The listing builds one solid part. Answer for the finished solid, in the listing's coordinates (mm). Coordinates: 2 decimals unless noted, no trailing zeros. Order: outer loops, then holes, each group sorted by start corner. A loop starts at its lowest first (then second) coordinate and runs counter-clockwise, first axis right, second up. Notation, with made-up numbers: (-23.75, 62.5) -> (-10.75, 62.5) arc R4 ccw to (-10.75, 67.5) -> close; hole circle Ø5 at (-15, 24). An arc over 180 degrees is marked (long way). Answer in a Markdown table with one row per item.
```python
from build123d import *

# Parameters (mm, degrees)
F1_DEPTH = 30


with BuildPart() as f1:
    # F0 (on Top) → F1 (new body)
    with BuildSketch(Plane.XY):
        with BuildLine():
            Line((17.858347, -1.59188), (0, -1.59188))
            Line((0, -1.59188), (0, -17.782362))
            Line((0, -17.782362), (2.289595, -17.782362))
            ThreePointArc((2.289595, -17.782362), (12.923538, -12.427261), (17.858347, -1.59188))
        make_face()
        with BuildLine():
            Line((24.029288, -1.59188), (17.858347, -1.59188))
            ThreePointArc((17.858347, -1.59188), (12.923538, -12.427261), (2.289595, -17.782362))
            Line((2.289595, -17.782362), (24.029288, -17.782362))
            Line((24.029288, -17.782362), (24.029288, -1.59188))
        make_face()
        with BuildLine():
            Line((0, -17.782362), (0, -1.59188))
            Line((0, -1.59188), (17.858347, -1.59188))
            ThreePointArc((17.858347, -1.59188), (17.911445, -0.796727), (17.929156, 0))
            ThreePointArc((17.929156, 0), (-13.463008, 11.840696), (2.289595, -17.782362))
            Line((2.289595, -17.782362), (0, -17.782362))
        make_face()
    extrude(amount=F1_DEPTH)


solid = f1.part
```
(1) For a pull along Y with two mould halves and no side action, classify faces 1 (the flat face through (13, -17.782, 15)), 2 (the flat face through (3, 0, 0)), 3 (the cylindrical face through (-13.054, 12.29, 14.79)), 4 (the cylindrical face through (17.91, -0.81, 14.79)) as released by +Y, released by -Y, zero draft, split by the parting line, or undercut.
Check values:
| item | result |
|---|---|
| face 1 | released by -Y |
| face 2 | zero draft |
| face 3 | split by the parting line |
| face 4 | undercut |
(2) Flat-ended cylindrical pins translate along their axes: pin 1 (6 mm diameter, centred on x = -6.5, z = 23.5, fed in from +Y); pin 2 (2 mm diameter, centred on x = -4.5, y = -3.5, fed in from -Z); pin 3 (17.5 mm diameter, centred on x = 14.5, z = 18, fed in from -Y); pin 4 (1 mm diameter, centred on x = -3.5, z = 16, fed in from +Y). Find the tip coordinate at first contact, or state that the pin passes through.
Check values:
| item | result |
|---|---|
| pin 1 | y = 17.58 |
| pin 2 | z = 0 |
| pin 3 | y = -17.78 |
| pin 4 | y = 17.68 |
(3) A cutting plane is placed at B-B, the plane x = 15. Determine the outline of the cut face in (y, z).
Check values:
| item | result |
|---|---|
| outline | (-17.78, 0) -> (9.82, 0) -> (9.82, 30) -> (-17.78, 30) -> close |
(4) A cutting plane is placed at A-A, the plane z = 19.5. Determine the outline of the cut face in (x, y), then the cut area to 3 significant figures.
Check values:
| item | result |
|---|---|
| outline | (2.29, -17.78) -> (24.03, -17.78) -> (24.03, -1.59) -> (17.86, -1.59) arc R17.93 ccw to (17.93, 0) arc R17.93 ccw (long way) to start |
| area | 1,180 mm² |
(5) A cutting plane is placed at C-C, the plane y = 9. Determine the outline of the cut face in (x, z), then the cut area to 3 significant figures.
Check values:
| item | result |
|---|---|
| outline | (-15.51, 0) -> (15.51, 0) -> (15.51, 30) -> (-15.51, 30) -> close |
| area | 930 mm² |
(6) Find the intervals of material crossed by line 1 along Y through (x, z) = (18, 2); line 2 along X through (y, z) = (13.5, 4); line 3 along X through (y, z) = (1.5, 8), in increasing order. Write a range as from..to.
Check values:
| item | result |
|---|---|
| line 1 | -17.78..-1.59 |
| line 2 | -11.8..11.8 |
| line 3 | -17.87..17.87 |
